from build123d import *

# Parameters (mm, degrees)
SKETCH4_R               = 1.3589
CUT_EXTRUDE1_DEPTH      = 5.7625
CUT_EXTRUDE1_DEPTH_BACK = 5.7625


with BuildPart() as part:
    # Sketch3 → Revolve1 (revolve)
    with BuildSketch(Plane.XY):
        Polygon((-6.35, 4.7625), (-6.35, 3.175), (0, 3.175), (0, 1.8923), (7.9502, 1.8923), (7.9502, 4.7625), align=None)
    revolve(axis=Axis((0, 0, 0), (1, 0, 0)))

    # Sketch4 → Cut-Extrude1 (cut, two sides)
    with BuildSketch(Plane(origin=(0, 0, 0), x_dir=(1, 0, 0), z_dir=(0, 1, 0))) as cut_extrude1_sk:
        with Locations((3.9624, 0)):
            Circle(SKETCH4_R)
    extrude(amount=CUT_EXTRUDE1_DEPTH, mode=Mode.SUBTRACT)
    extrude(cut_extrude1_sk.sketch, amount=-CUT_EXTRUDE1_DEPTH_BACK, mode=Mode.SUBTRACT)


solid = part.part
Can you work these out from the model? Positions are in its coordinate system, mm. A direction names the side the tool comes from. Give positions to 0.01 mm unless a question says otherwise; leave off trailing zeros. Loops run counter-clockwise (first coordinate to the right, second up) from the corner with the lowest first, then second, coordinate; pieces in that order, holes last. Notation, with made-up numbers: M 73.5,-34.5 L 98.5,-34.5 A31 cw 98.5,-0.5 Z; hole C -33,-19 d10. An arc over 180 degrees is marked long. One line per item, written item: value.
1) Imagine slicing it at A-A on z = 0. Count the separate pieces of the cut face and the enclosed holes in it, and give its area (3 significant figures).
Geometry check:
separate pieces: 4
enclosed holes: 0
area: 50.2 mm²
2) Thinking about a two-plate mould opening in Y: for faces 3 (the face through (4.031, -0.41, -1.847)), 4 (the face through (-3.13, -0.69, -3.1)), 5 (the face through (5.22, -3.02, 0.52)), 6 (the face through (0.7, 4.543, 1.431)), which applies, +Y half, -Y half, draft (parallel to the pull), parting line (faces both ways), or undercut?
Geometry check:
face 3: undercut
face 4: undercut
face 5: draft
face 6: parting line
3) I'm going to push flat-ended pins straight in: pin 1 (2 mm diameter, centred on x = 0, z = 2.5, fed in from -Y); pin 2 (2 mm diameter, centred on x = 4, z = -2, fed in from -Y); pin 3 (1.9 mm diameter, centred on y = -1.5, z = 1.5, fed in from -X). Where does each tip first touch, or does it pass through?
Geometry check:
pin 1: stops at y = -4.52
pin 2: stops at y = -4.61
pin 3: stops at x = 0
4) Please list where these lines run through material, in increasing order: line 1 (Y direction, x = 6, z = 0); line 2 (Z direction, x = -1.75, y = 0) (1 decimal).
Geometry check:
line 1: y = -4.76 to -1.89, 1.89 to 4.76
line 2: z = -4.8 to -3.2, 3.2 to 4.8
5) Imagine slicing it at C-C on x = 3.5. Write out the boundary of the cut face in (y, z) (1 decimal).
Geometry check:
outline: M -4.6,-1.3 A4.8 ccw 4.6,-1.3 L 1.4,-1.3 A1.9 cw -1.4,-1.3 Z; M -4.6,1.3 L -1.4,1.3 A1.9 cw 1.4,1.3 L 4.6,1.3 A4.8 ccw Z
6) Imagine slicing it at D-D on y = 3. Write out the boundary of the cut face in (x, z), and give its area (3 significant figures).
Geometry check:
outline: M -6.35,-3.7 L 7.95,-3.7 L 7.95,3.7 L -6.35,3.7 L -6.35,1.04 L 0,1.04 L 0,-1.04 L -6.35,-1.04 Z; hole C 3.96,0 d2.72
area: 86.8 mm²
7) On a 3-axis mill with a long thin cutter (end or side, diameter ignored), from which of +Z, -Z, +X, -X, +Y, -Y can I reach the whole of each face in a straight line? I mean faces 1 (the face through (7.95, -2.05, 0.07)), 2 (the face through (0, 0, -2.1)). Say none if no direction works.
Geometry check:
face 1: +Z, -Z, +X, +Y, -Y
face 2: -X
